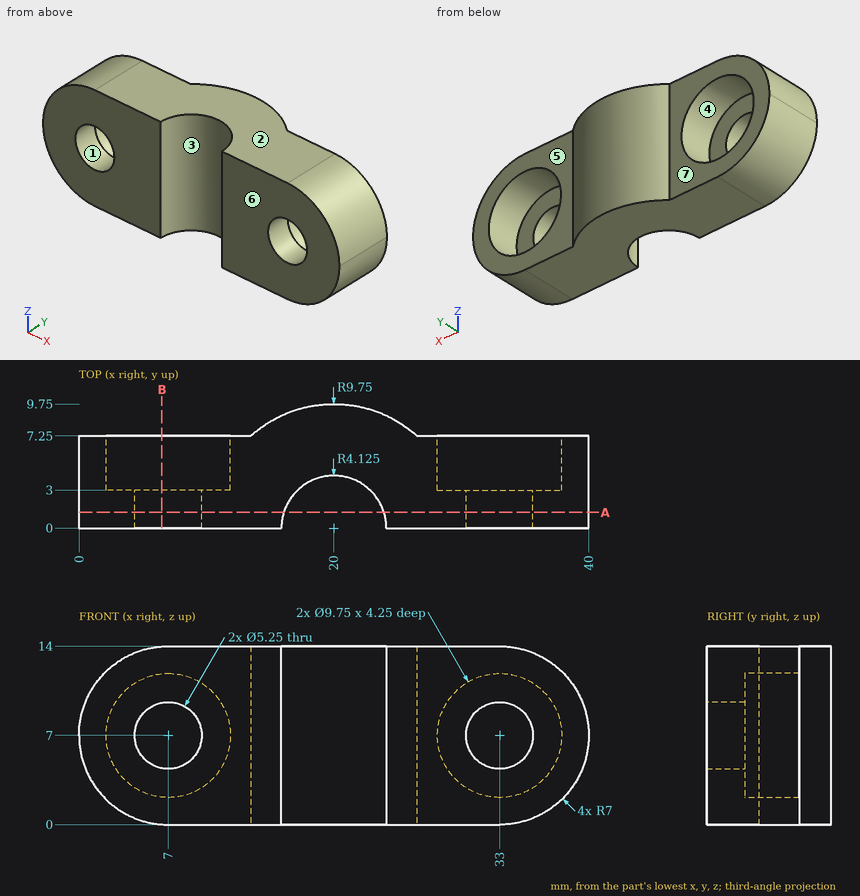
Study the drawing (mm; zero at the part's minimum x, y, z) and answer. A direction names the side the tool comes from. Give positions to 0.01 mm unless a question says otherwise; leave off trailing zeros. Loops run counter-clockwise (first coordinate to the right, second up) from the corner with the lowest first, then second, coordinate; pieces in that order, holes last. Notation, with made-up numbers: (57, 42.25) - (113, 42.25) arc R26 cw to (113, 66.25) - close; hole circle Ø11 at (-40, -21.5). An arc over 180 degrees is marked (long way). One line per question, with ' | ' between items.
(1) The part is cut by section B-B (x = 6.5). Write down the section's boundary in (y, z), then the cut area to 3 significant figures.
Recorded:
outline: (0, 0.02) - (7.25, 0.02) - (7.25, 2.15) - (3, 2.15) - (3, 4.42) - (0, 4.42) - close; (0, 9.58) - (3, 9.58) - (3, 11.85) - (7.25, 11.85) - (7.25, 13.98) - (0, 13.98) - close | area: 44.6 mm²
(2) The mould has two halves that part along Z. Classify the marked faces 1, 2 and 3: +Z half, -Z half, draft (parallel to the pull), parting line (faces both ways), or undercut.
Recorded:
face 1: undercut | face 2: +Z half | face 3: draft
(3) Straight lines are drawn through the part: probe 1 along X at (y, z) = (6.3, 7) (3 decimals); probe 2 along X at (y, z) = (5.5, 4.25) (1 decimal); probe 3 along X at (y, z) = (0.7, 7) (3 decimals). For each, find the intervals that lie inside material, in ascending order.
Recorded:
probe 1: x = 0 to 2.125, 11.875 to 28.125, 37.875 to 40 | probe 2: x = 0.6 to 3, 11 to 29, 37 to 39.4 | probe 3: x = 0 to 4.375, 9.625 to 15.935, 24.065 to 30.375, 35.625 to 40
(4) A tool of negligible diameter and unlimited length cuts with its end or side. For the marked faces 4, 5, 6 and 7, from which of +Z, -Z, +X, -X, +Y, -Y can it reach the whole face along a straight path? Write none if from no direction.
Recorded:
face 4: +Y | face 5: +Z, -Z, +X, +Y | face 6: +Z, -Z, +X, -X, -Y | face 7: +Z, -Z, -X, +Y
(5) Each of these flat-tipped pins is pushed along its axis until it touches: pin 1 Ø3 at (x, y) = (34, 6) entering from -Z; pin 2 Ø5 at (x, z) = (31.5, 7) entering from +Y; pin 3 Ø6.5 at (x, z) = (5.5, 9.5) entering from +Y; pin 4 Ø2 at (x, z) = (22.5, 12) entering from -Y. Where does it stop, or does it pass through?
Recorded:
pin 1: stops at z = 0 | pin 2: stops at y = 3 | pin 3: stops at y = 7.25 | pin 4: stops at y = 2.18
(6) The part is cut by section A-A (y = 1.25). Count the separate pieces of the cut face and the enclosed holes in it, then the cut area to 3 significant figures.
Recorded:
separate pieces: 2 | enclosed holes: 2 | area: 365 mm²
